Design review of the part built by this model. Coordinates are the model's own, in mm. Face numbers are marked on the shaded views. A direction names the side the tool comes from. Round coordinates to 2 decimals unless told otherwise and drop trailing zeros. Loops run counter-clockwise (first coordinate to the right, second up) from the corner with the lowest first, then second, coordinate; pieces in that order, holes last. Notation, with made-up numbers: (38.25, 78.5) - (55.25, 78.5) arc R19 ccw to (55.25, 87.5) - close; hole circle Ø10 at (11.25, -21.5). An arc over 180 degrees is marked (long way). Answer as CSV lines item,"result". Start each with the question number.
(1) Wall thickness on L1, parallel to Y at x = -32, z = 6.75; L2, parallel to Y at x = -22, z = 8; L3, parallel to Y at x = -32, z = 7.5: over which ranges is each line inside the solid? List them lowest first.
(2) Consider section D-D (x = -18.5). Give the boundary of the cut face in (y, z), and give its area (3 significant figures).
(3) For the marked faces 5 and 6, list the 3-axis set-ups (+Z, -Z, +X, -X, +Y, -Y) from which the entire face can be reached by the end or side of a thin tool; tool diameter is ignored.
(4) Mouldability with a two-part tool opening along X and no side actions: class the marked faces 1, 2, 3 and 4 as released by +X, released by -X, zero draft, split by the parting line, or undercut.
(5) For P1, Ø2, axis at x = -38, y = 5.5, coming from the +Z side; P2, Ø5, axis at y = -11.5, z = 5.5, coming from the +X side; P3, Ø3, axis at y = -2, z = 2.5, coming from the +X side; P4, Ø6, axis at x = 4.5, y = 13.5, coming from the +Z side, all flat-tipped, find the tip position at first contact; note any pin that passes through.
(6) Consider section B-B (z = 13.25). Give the boundary of the cut face in (x, y), and give its area (3 significant figures).
(7) Consider section A-A (x = 6). Give the boundary of the cut face in (y, z).
(8) Consider section C-C (y = -14). Give the boundary of the cut face in (x, z), and give its area (3 significant figures).
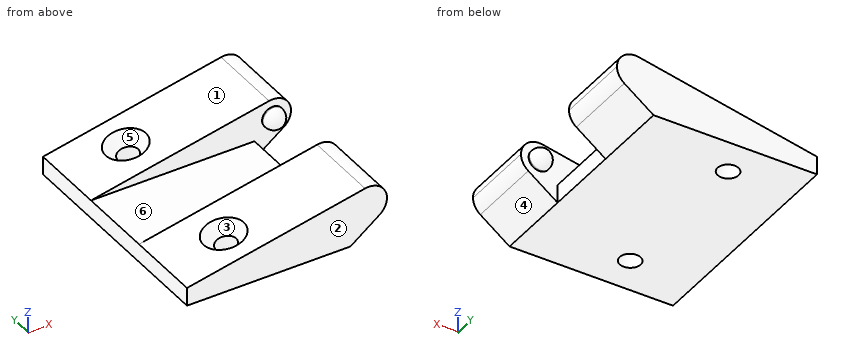
from build123d import *

# Parameters (mm, degrees)
F0_W            = 53.6510385573
F0_H            = 6
F0_R            = 3
F1_DEPTH        = 37.5
F1_DEPTH_BACK   = 37.5
F3_DEPTH        = 12.5
F3_DEPTH_BACK   = 12.5
F4_R            = 3.5
F5_DEPTH        = 4
F6_R            = 3.5
F7_DEPTH        = 4
F8_R            = 3.5
F10_D           = 6.7564
F10_CSINK_D     = 13.4874
F10_CSINK_ANGLE = 82


# Not quite as in the source:
# - a feature of the source that left no trace in its solid (it failed there, or was rolled back) is left out


with BuildPart() as f1:
    # F0 (on Front) → F1 (new body, two sides)
    with BuildSketch(Plane.XZ) as f1_sk:
        with Locations((-26.8255192786, 3)):
            Rectangle(F0_W, F0_H)
        with BuildLine():
            Line((0, 6), (0, 0))
            Line((0, 0), (9.6, 7.2))
            ThreePointArc((9.6, 7.2), (0.5263664708, 9.5424939495), (4.8050694646, 17.8798079064))
            Line((4.8050694646, 17.8798079064), (-53.6510385573, 6))
            Line((-53.6510385573, 6), (0, 6))
        make_face()
        with BuildLine():
            ThreePointArc((4.8050694646, 17.8798079064), (0.5263664708, 9.5424939495), (9.6, 7.2))
            ThreePointArc((9.6, 7.2), (11.366563146, 9.316718427), (12, 12))
            ThreePointArc((12, 12), (9.7967365452, 16.6459435647), (4.8050694646, 17.8798079064))
        make_face()
        with Locations((6, 12)):
            Circle(F0_R, mode=Mode.SUBTRACT)
        with Locations((6, 12)):
            Circle(F0_R)
    extrude(amount=F1_DEPTH)
    extrude(f1_sk.sketch, amount=-F1_DEPTH_BACK)

    # F0 (on Front) → F3 (cut, two sides)
    with BuildSketch(Plane.XZ) as f3_sk:
        with BuildLine():
            Line((0, 6), (0, 0))
            Line((0, 0), (9.6, 7.2))
            ThreePointArc((9.6, 7.2), (0.5263664708, 9.5424939495), (4.8050694646, 17.8798079064))
            Line((4.8050694646, 17.8798079064), (-53.6510385573, 6))
            Line((-53.6510385573, 6), (0, 6))
        make_face()
        with BuildLine():
            ThreePointArc((4.8050694646, 17.8798079064), (0.5263664708, 9.5424939495), (9.6, 7.2))
            ThreePointArc((9.6, 7.2), (11.366563146, 9.316718427), (12, 12))
            ThreePointArc((12, 12), (9.7967365452, 16.6459435647), (4.8050694646, 17.8798079064))
        make_face()
        with Locations((6, 12)):
            Circle(F0_R, mode=Mode.SUBTRACT)
        with Locations((6, 12)):
            Circle(F0_R)
    extrude(amount=F3_DEPTH, mode=Mode.SUBTRACT)
    extrude(f3_sk.sketch, amount=-F3_DEPTH_BACK, mode=Mode.SUBTRACT)

    # F4 (on face) → F5 (join)
    with BuildSketch(Plane.XZ.offset(-12.5)):
        with Locations((6, 12)):
            Circle(F4_R)
    extrude(amount=F5_DEPTH)

    # F6 (on face) → F7 (join)
    with BuildSketch(Plane(origin=(0, -12.5, 0), x_dir=(-1, 0, 0), z_dir=(0, 1, 0))):
        with Locations((-6, 12)):
            Circle(F6_R)
    extrude(amount=F7_DEPTH)

    # F8
    f8_edges = [f1.edges().sort_by_distance(p)[0] for p in [
        (9.5, -8.5, 12),
        (2.5, 8.5, 12),
    ]]
    fillet(f8_edges, radius=F8_R)

    # F10 (through all)
    with Locations(Plane(origin=(-3.2989413744, 0, 16.2328612433), x_dir=(0.9799679844, 0, 0.1991550892), z_dir=(-0.1991550892, 0, 0.9799679844))):
        with Locations((-31.3813695802, -25.5), (-31.3813695802, 25.5)):
            CounterSinkHole(F10_D / 2, F10_CSINK_D / 2, counter_sink_angle=F10_CSINK_ANGLE)


solid = f1.part
Determined:
1,L1,"y = -37.5 to -28.87, -22.13 to -12.5, 12.5 to 22.13, 28.87 to 37.5"
1,L2,"y = -37.5 to -12.5, 12.5 to 37.5"
1,L3,"y = -37.5 to -29.5, -21.5 to -12.5, 12.5 to 21.5, 29.5 to 37.5"
2,outline,"(-37.5, 0) - (37.5, 0) - (37.5, 13.14) - (12.5, 13.14) - (12.5, 6) - (-12.5, 6) - (-12.5, 13.14) - (-37.5, 13.14) - close"
2,area,"807 mm^2"
3,face 5,"+Z"
3,face 6,"+Z, +X, -X"
4,face 1,"released by -X"
4,face 2,"zero draft"
4,face 3,"undercut"
4,face 4,"released by +X"
5,P1,"stops at z = 6"
5,P2,"stops at x = 10.28"
5,P3,"stops at x = 0"
5,P4,"stops at z = 18"
6,outline,"(-17.98, -37.5) - (11.87, -37.5) - (11.87, -12.5) - (9.27, -12.5) - (9.27, -12) arc R3.27 ccw to (2.73, -12) - (2.73, -12.5) - (-17.98, -12.5) - close; (-17.98, 12.5) - (2.73, 12.5) - (2.73, 12) arc R3.27 ccw to (9.27, 12) - (9.27, 12.5) - (11.87, 12.5) - (11.87, 37.5) - (-17.98, 37.5) - close"
6,area,"1,530 mm^2"
7,outline,"(-37.5, 4.5) - (-12.5, 4.5) - (-12.5, 8.5) - (-12, 8.5) arc R3.5 ccw to (-12, 15.5) - (-12.5, 15.5) - (-12.5, 18) - (-37.5, 18) - close; (12, 8.5) - (12.5, 8.5) - (12.5, 4.5) - (37.5, 4.5) - (37.5, 18) - (12.5, 18) - (12.5, 15.5) - (12, 15.5) arc R3.5 ccw to start"
8,outline,"(-53.65, 0) - (0, 0) - (9.6, 7.2) arc R6 ccw to (4.81, 17.88) - (-53.65, 6) - close"
8,area,"764 mm^2"
